Geometry check sheet. Reference: the model listing, model coordinates, mm. Face numbers are marked on the shaded views. A direction names the side the tool comes from. Round coordinates to 2 decimals unless told otherwise and drop trailing zeros. Order: outer loops, then holes, each group sorted by start corner. A loop starts at its lowest first (then second) coordinate and runs counter-clockwise, first axis right, second up. Notation, with made-up numbers: (58, -19.75) -> (68, -19.75) arc R20 ccw to (68, -13.75) -> close; hole circle Ø10 at (54, 4.25). An arc over 180 degrees is marked (long way). Use a Markdown table: item, result. Add a question column.
Item 1: Material ranges on probe 1 along X at (y, z) = (8.15, 0); probe 2 along Z at (x, y) = (-15, 8.1); probe 3 along X at (y, z) = (5.25, 0.75), recorded low to high. Write a range as [from, to].
Item 2: Sectioned sample at B-B, the plane y = 1. Record the cut outline in (x, z), and give its area (3 significant figures).
Item 3: Sectioned sample at C-C, the plane z = 0. Record the cut outline in (x, y).
Item 4: Sectioned sample at D-D, the plane y = 6.25. Record the cut outline in (x, z).
Item 5: Mould release check, pull along Z, two halves, no side actions. Record for the marked faces 1, 2 and 3: pulls with the +Z half, pulls with the -Z half, needs draft (parallel to the pull), parting line crosses it, or undercut.
Item 6: Sectioned sample at A-A, the plane x = 15. Record the cut outline in (y, z), and give its area (3 significant figures).
Item 7: Gauge pin test, flat ends, axial feed: pin 1 Ø2.5 at (x, z) = (15, 0) entering from -Y; pin 2 Ø5 at (x, z) = (-15, 0) entering from -Y; pin 3 Ø4 at (x, y) = (-14, 3.5) entering from +Z; pin 4 Ø4 at (x, y) = (17.5, 3) entering from -Z. Record the tip position at first contact, or that the pin passes through.
Item 8: Set-up check for the marked faces 4, 5, 6 and 7: record each of +Z, -Z, +X, -X, +Y, -Y from which the full face is reachable in a straight line by a thin tool's end or side.
Autodesk Inventor part; units mm, degrees
ref_plane "YZ Plane" through (0, 0, 0) normal (1, 0, 0) x (0, 1, 0)
ref_plane "XZ Plane" through (0, 0, 0) normal (0, 1, 0) x (-1, 0, 0)
ref_plane "XY Plane" through (0, 0, 0) normal (0, 0, 1) x (1, 0, 0)
sketch "Эскиз1" plane through (0, 0, 0) normal (0, 1, 0) x (-1, 0, 0)
  circle A0 centre (0, 0) radius 5
  line L0 (8, 10) -> (-8, 10)
  line L1 (-10, 8) -> (-10, -8)
  line L2 (-8, -10) -> (8, -10)
  line L3 (10, -8) -> (10, 8)
  circle A1 centre (0, 0) radius 8 construction
  line L4 (8, 10) -> (10, 8)
  line L5 (10, -8) -> (8, -10)
  line L6 (-8, -10) -> (-10, -8)
  line L7 (-8, 10) -> (-10, 8)
  point P0 (10, 10)
  point P1 (-10, -10)
  point P2 (-10, 10)
  point P3 (10, -10)
  point P4 (0, -10)
  point P5 (10, 0)
  dimension "d0" = 10
  dimension "d3" = 16
  dimension "d4" = 20
  dimension "d5" = 20
  dimension "d6" = 2
  dimension "d7" = 2
  dimension "d8" = 2
  dimension "d9" = 2
  dimension "d10" = 2
  dimension "d11" = 2
  dimension "d12" = 2
  dimension "d13" = 2
extrude "Выдавливание1" add sketch "Эскиз1" along normal blind 5
sketch "Эскиз4" plane through (0, 5, 0) normal (0, 1, 0) x (1, 0, 0)
  line L0 (12.8246, 0) -> (14.4123, 2.75) construction
  line L1 (14.4123, 2.75) -> (17.5877, 2.75) construction
  line L2 (17.5877, 2.75) -> (19.1754, 0) construction
  line L3 (19.1754, 0) -> (17.5877, -2.75) construction
  line L4 (17.5877, -2.75) -> (14.4123, -2.75) construction
  line L5 (14.4123, -2.75) -> (12.8246, 0) construction
  line L6 (10, -8) -> (20, -8)
  line L7 (20, -8) -> (20, 8)
  line L8 (20, 8) -> (10, 8)
  line L9 (8, -10) -> (10, -8)
  line L10 (10, -8) -> (8, -10)
  line L11 (8, -10) -> (0, -10)
  line L12 (8, -10) -> (-8, -10)
  line L13 (8, 10) -> (0, 10)
  line L14 (8, 10) -> (-8, 10)
  line L15 (10, 8) -> (8, 10)
  line L16 (10, 8) -> (8, 10)
  line L17 (0, -18.8546) -> (0, 18.8546)
  line L18 (-12.8246, 0) -> (-14.4123, 2.75) construction
  line L19 (-14.4123, 2.75) -> (-17.5877, 2.75) construction
  line L20 (-17.5877, 2.75) -> (-19.1754, 0) construction
  line L21 (-19.1754, 0) -> (-17.5877, -2.75) construction
  line L22 (-17.5877, -2.75) -> (-14.4123, -2.75) construction
  line L23 (-14.4123, -2.75) -> (-12.8246, 0) construction
  line L24 (-10, -8) -> (-20, -8)
  line L25 (-20, -8) -> (-20, 8)
  line L26 (-20, 8) -> (-10, 8)
  line L27 (-8, -10) -> (-10, -8)
  line L28 (-10, -8) -> (-8, -10)
  line L29 (-8, -10) -> (0, -10)
  line L30 (-8, 10) -> (0, 10)
  line L31 (-10, 8) -> (-8, 10)
  line L32 (-10, 8) -> (-8, 10)
  point P0 (0, 0)
  point P1 (16, 0)
  point P2 (0, 0)
  point P3 (-16, 0)
  dimension "d17" = 5.5
  dimension "d18" = 16
  dimension "d19" = 10
extrude "Выдавливание2" add sketch "Эскиз4" along normal blind 4
sketch "Эскиз7" plane through (0, 9, 0) normal (0, 1, 0) x (1, 0, 0)
  circle A0 centre (0, 0) radius 8.1
  dimension "d26" = 16.2
extrude "Выдавливание4" cut sketch "Эскиз7" against normal blind 7
sketch "Эскиз10" plane through (-10, 5, -8) normal (0, 0, -1) x (-1, 0, 0)
  line L0 (10, 0) -> (10, 4)
  line L1 (-2, -5) -> (0, -5)
  line L2 (10, 0) -> (0, -5)
  line L3 (0, -5) -> (0, 0)
  line L4 (10, 0) -> (0, 0)
  line L5 (0, 0) -> (10, 0)
  point P0 (-10, -5)
extrude "Выдавливание5" add sketch "Эскиз10" against normal blind 3
mirror "Зеркальное отражение1" about plane through (0, 0, 0) normal (0, 0, 1) of "Выдавливание5"
mirror "Зеркальное отражение2" about plane through (0, 0, 0) normal (1, 0, 0) of "Выдавливание5", "Зеркальное отражение1"
chamfer "Фаска1" distance 2 angle 45 4 edges at (-20, 7, -8) (20, 7, -8) (20, 7, 8) (-20, 7, 8)
sketch "Эскиз11" plane through (0, 5, 0) normal (0, -1, 0) x (1, 0, 0)
  point P0 (0, 0)
  point P1 (15, 0)
  point P2 (-15, 0)
  dimension "d48" = 30
  dimension "d49" = 15
hole "Отверстие2" at (15, 5, 0) at (-15, 5, 0) direction (0, 1, 0) diameter 3.2 end through all
properties part number "Sharrnir"
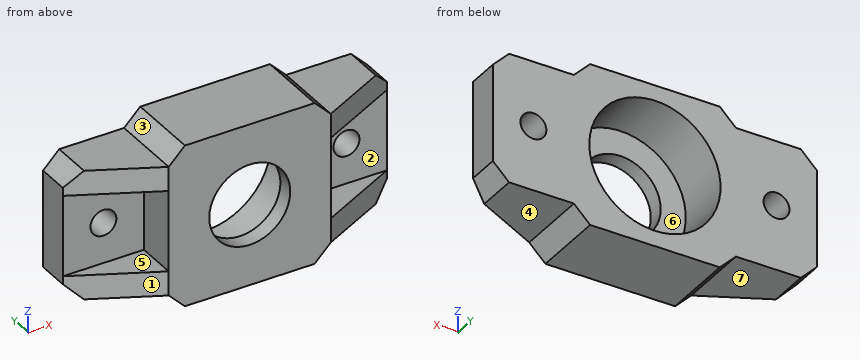
Found:
| question | item | result |
|---|---|---|
| 1 | probe 1 | x = [-20, -16.6], [-13.4, -8.1], [8.1, 13.4], [16.6, 20] |
| 1 | probe 2 | z = [-8, -1.6], [1.6, 8] |
| 1 | probe 3 | x = [-20, -16.41], [-13.59, -8.07], [8.07, 13.59], [16.41, 20] |
| 2 | outline | (-12, -8) -> (-10, -8) -> (-8, -10) -> (8, -10) -> (10, -8) -> (12, -8) -> (12, -5) -> (10, -5) -> (10, 5) -> (12, 5) -> (12, 8) -> (10, 8) -> (8, 10) -> (-8, 10) -> (-10, 8) -> (-12, 8) -> (-12, 5) -> (-10, 5) -> (-10, -5) -> (-12, -5) -> close; hole circle Ø10 at (0, 0) |
| 2 | area | 337 mm2 |
| 3 | outline | (-20, 5) -> (-16.6, 5) -> (-16.6, 9) -> (-20, 9) -> close; (-13.4, 5) -> (-10, 5) -> (-10, 0) -> (-5, 0) -> (-5, 2) -> (-8.1, 2) -> (-8.1, 9) -> (-13.4, 9) -> close; (5, 0) -> (10, 0) -> (10, 5) -> (13.4, 5) -> (13.4, 9) -> (8.1, 9) -> (8.1, 2) -> (5, 2) -> close; (16.6, 5) -> (20, 5) -> (20, 9) -> (16.6, 9) -> close |
| 4 | outline | (-20, -6) -> (-18, -8) -> (-10, -8) -> (-8, -10) -> (8, -10) -> (10, -8) -> (18, -8) -> (20, -6) -> (20, 6) -> (18, 8) -> (10, 8) -> (8, 10) -> (-8, 10) -> (-10, 8) -> (-18, 8) -> (-20, 6) -> close; hole circle Ø3.2 at (-15, 0); hole circle Ø16.2 at (0, 0); hole circle Ø3.2 at (15, 0) |
| 5 | face 1 | needs draft |
| 5 | face 2 | undercut |
| 5 | face 3 | pulls with the +Z half |
| 6 | outline | (2.5, -8) -> (9, -8) -> (9, -1.6) -> (5, -1.6) -> (5, -5) -> (2.5, -5) -> close; (2.5, 5) -> (5, 5) -> (5, 1.6) -> (9, 1.6) -> (9, 8) -> (2.5, 8) -> close |
| 6 | area | 66.2 mm2 |
| 7 | pin 1 | passes through |
| 7 | pin 2 | stops at y = 5 |
| 7 | pin 3 | stops at z = 8 |
| 7 | pin 4 | stops at z = -8 |
| 8 | face 4 | -Z, +X, +Y, -Y |
| 8 | face 5 | -X, -Y |
| 8 | face 6 | +Y |
| 8 | face 7 | -Z, -X, +Y, -Y |
